Geometry check sheet. Reference: drawing and pictorial views, mm from the part's lowest x, y, z. Coordinates: 2 decimals unless noted, no trailing zeros. Loops run counter-clockwise (first coordinate to the right, second up) from the corner with the lowest first, then second, coordinate; pieces in that order, holes last.
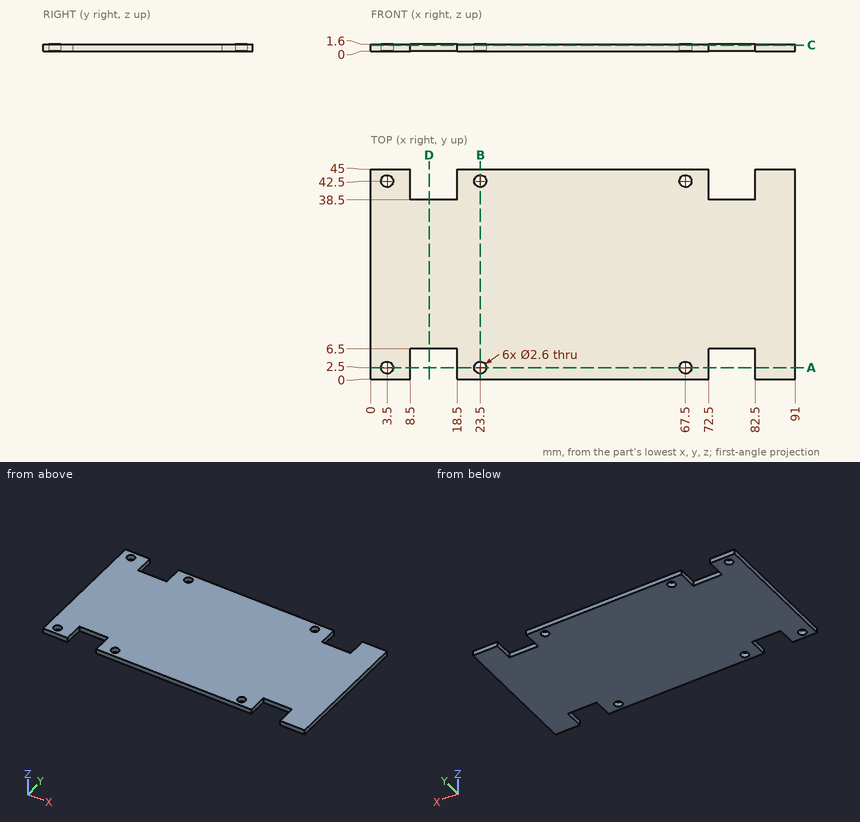
1) Section check B-B on x = 23.5. Record the cut outline in (y, z), and give its area (3 significant figures).
Data:
outline: (0, 0) - (1.2, 0) - (1.2, 1.6) - (0, 1.6) - close; (3.8, 0) - (41.2, 0) - (41.2, 1.6) - (3.8, 1.6) - close; (43.8, 0) - (45, 0) - (45, 1.6) - (43.8, 1.6) - close
area: 63.7 mm2
2) Section check D-D on x = 12.5. Record the cut outline in (y, z), and give its area (3 significant figures).
Data:
outline: (6.5, 0) - (38.5, 0) - (38.5, 1.6) - (6.5, 1.6) - close
area: 51.2 mm2
3) Material ranges on probe 1 along Y at (x, z) = (67.5, 1.2); probe 2 along X at (y, z) = (42.5, 1.05); probe 3 along Y at (x, z) = (4, 0.1), recorded low to high.
Data:
probe 1: y = 0 to 1.2, 3.8 to 41.2, 43.8 to 45
probe 2: x = 0 to 2.2, 4.8 to 8.5, 18.5 to 22.2, 24.8 to 66.2, 68.8 to 72.5, 82.5 to 91
probe 3: y = 0 to 1.3, 3.7 to 41.3, 43.7 to 45
4) Section check A-A on y = 2.5. Record the cut outline in (x, z), and give its area (3 significant figures).
Data:
outline: (0, 0) - (2.2, 0) - (2.2, 1.6) - (0, 1.6) - close; (4.8, 0) - (8.5, 0) - (8.5, 1.6) - (4.8, 1.6) - close; (18.5, 0) - (22.2, 0) - (22.2, 1.6) - (18.5, 1.6) - close; (24.8, 0) - (66.2, 0) - (66.2, 1.6) - (24.8, 1.6) - close; (68.8, 0) - (72.5, 0) - (72.5, 1.6) - (68.8, 1.6) - close; (82.5, 0) - (91, 0) - (91, 1.6) - (82.5, 1.6) - close
area: 101 mm2
5) Section check C-C on z = 1.35. Record the cut outline in (x, y).
Data:
outline: (0, 0) - (8.5, 0) - (8.5, 6.5) - (18.5, 6.5) - (18.5, 0) - (72.5, 0) - (72.5, 6.5) - (82.5, 6.5) - (82.5, 0) - (91, 0) - (91, 45) - (82.5, 45) - (82.5, 38.5) - (72.5, 38.5) - (72.5, 45) - (18.5, 45) - (18.5, 38.5) - (8.5, 38.5) - (8.5, 45) - (0, 45) - close; hole circle Ø2.6 at (3.5, 2.5); hole circle Ø2.6 at (3.5, 42.5); hole circle Ø2.6 at (23.5, 2.5); hole circle Ø2.6 at (23.5, 42.5); hole circle Ø2.6 at (67.5, 2.5); hole circle Ø2.6 at (67.5, 42.5)
6) Depth check by flat-ended pin: pin 1 (2.5 mm diameter, centred on x = 3.5, y = 42.5, fed in from +Z); pin 2 (0.5 mm diameter, centred on x = 79.5, z = 1, fed in from +Y); pin 3 (0.5 mm diameter, centred on x = 15.5, z = 1, fed in from -Y). Enter the tip coordinate at first touch or a pass-through.
Data:
pin 1: passes through
pin 2: stops at y = 38.5
pin 3: stops at y = 6.5
